Here's the drawing with two shaded views (mm, measured from the low corner). I have some questions. A direction names the side the tool comes from. Give positions to 0.01 mm unless a question says otherwise; leave off trailing zeros. Write each loop counter-clockwise with the first axis right and the second up, starting at its lowest first coordinate (ties: lowest second). Pieces come first, ordered by that corner, then holes. Notation, with made-up numbers: (18.25, 1.25) -> (28.25, 1.25) arc R13 cw to (28.25, 12.25) -> close; hole circle Ø10 at (65, 71.25). An arc over 180 degrees is marked (long way). One line per item, written item: value.
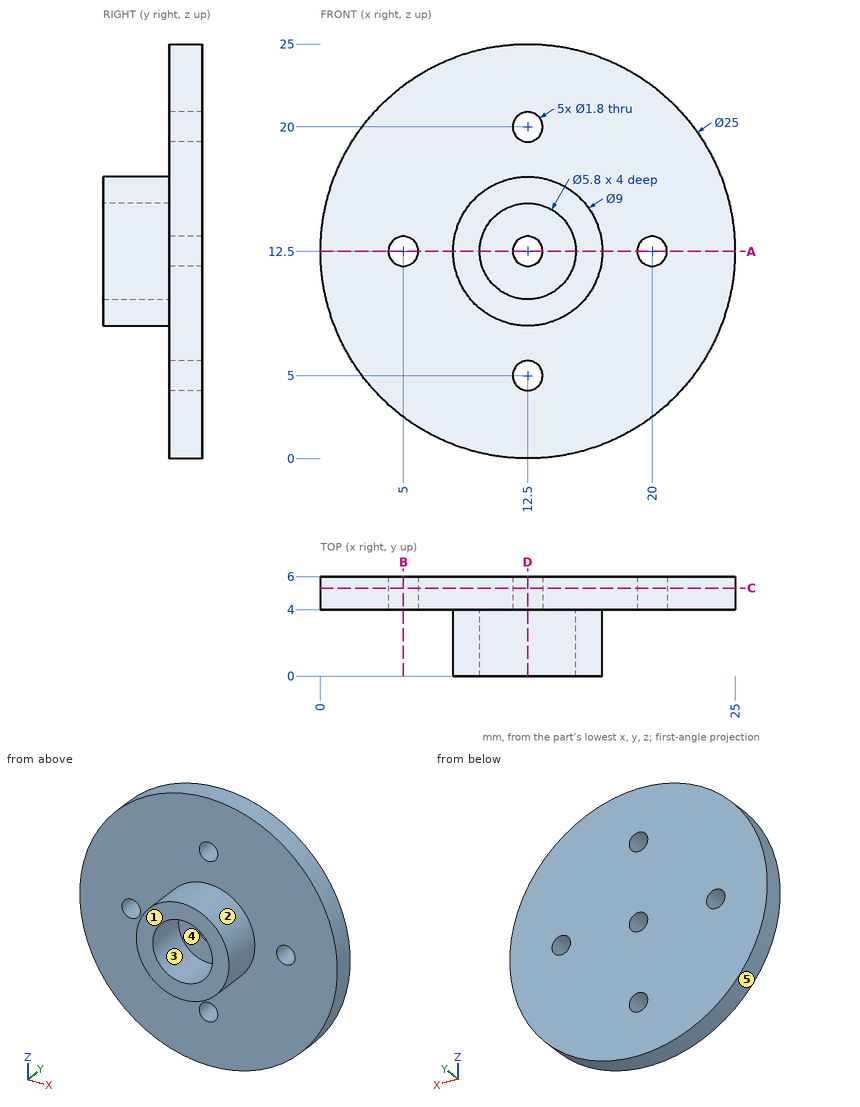
1) If we section it at C-C (y = 5.3): Write out the boundary of the cut face in (x, z).
Answer list:
outline: circle Ø25 at (12.5, 12.5); hole circle Ø1.8 at (5, 12.5); hole circle Ø1.8 at (12.5, 5); hole circle Ø1.8 at (12.5, 12.5); hole circle Ø1.8 at (12.5, 20); hole circle Ø1.8 at (20, 12.5)
2) If we section it at A-A (z = 12.5): Write out the boundary of the cut face in (x, y), and give its area (3 significant figures).
Answer list:
outline: (0, 4) -> (4.1, 4) -> (4.1, 6) -> (0, 6) -> close; (5.9, 4) -> (8, 4) -> (8, 0) -> (9.6, 0) -> (9.6, 4) -> (11.6, 4) -> (11.6, 6) -> (5.9, 6) -> close; (13.4, 4) -> (15.4, 4) -> (15.4, 0) -> (17, 0) -> (17, 4) -> (19.1, 4) -> (19.1, 6) -> (13.4, 6) -> close; (20.9, 4) -> (25, 4) -> (25, 6) -> (20.9, 6) -> close
area: 52.0 mm^2
3) We'd pull the mould along Z, two halves only. Please class the marked faces 1, 2 and 3: released by +Z, released by -Z, zero draft, split by the parting line, or undercut.
Answer list:
face 1: zero draft
face 2: split by the parting line
face 3: undercut
4) If we section it at D-D (x = 12.5): Write out the boundary of the cut face in (y, z), and give its area (3 significant figures).
Answer list:
outline: (0, 8) -> (4, 8) -> (4, 5.9) -> (6, 5.9) -> (6, 11.6) -> (4, 11.6) -> (4, 9.6) -> (0, 9.6) -> close; (0, 15.4) -> (4, 15.4) -> (4, 13.4) -> (6, 13.4) -> (6, 19.1) -> (4, 19.1) -> (4, 17) -> (0, 17) -> close; (4, 0) -> (6, 0) -> (6, 4.1) -> (4, 4.1) -> close; (4, 20.9) -> (6, 20.9) -> (6, 25) -> (4, 25) -> close
area: 52.0 mm^2
5) If we section it at B-B (x = 5): Write out the boundary of the cut face in (y, z), and give its area (3 significant figures).
Answer list:
outline: (4, 2.5) -> (6, 2.5) -> (6, 11.6) -> (4, 11.6) -> close; (4, 13.4) -> (6, 13.4) -> (6, 22.5) -> (4, 22.5) -> close
area: 36.4 mm^2
6) For the marked faces 4 and 5, which set-ups out of +Z, -Z, +X, -X, +Y, -Y let a thin tool reach every point of the face, with its end or its side?
Answer list:
face 4: -Y
face 5: +Y, -Y
7) Will these pins go through, and if not, where does the flat tip stop? pin 1 (12.5 mm diameter, centred on x = 13.5, z = 9.5, fed in from -Y); pin 2 (4.5 mm diameter, centred on x = 12.5, z = 12.5, fed in from -Y); pin 3 (1 mm diameter, centred on y = 4, z = 14.5, fed in from +X); pin 4 (1 mm diameter, centred on y = 1.5, z = 14, fed in from +X).
Answer list:
pin 1: stops at y = 0
pin 2: stops at y = 4
pin 3: stops at x = 24.91
pin 4: stops at x = 16.89
8) I need wall thicknesses on L1, parallel to X at y = 4.6, z = 12.5; L2, parallel to Y at x = 5, z = 20.25; L3, parallel to X at y = 4.9, z = 5. Which ranges of each line are inside material? Lowest first, please.
Answer list:
L1: x = 0 to 4.1, 5.9 to 11.6, 13.4 to 19.1, 20.9 to 25
L2: y = 4 to 6
L3: x = 2.5 to 11.6, 13.4 to 22.5
